from build123d import *

# Parameters (mm, degrees)
F1_DEPTH = 5


with BuildPart() as f1:
    # F0 (on Top) → F1 (new body)
    with BuildSketch(Plane.XY):
        with BuildLine():
            Line((23.528581, 23.329832), (-26.471419, 23.329832))
            Line((-26.471419, 23.329832), (-26.471419, 1.829832))
            ThreePointArc((-26.471419, 1.829832), (-26.032079, 0.769172), (-24.971419, 0.329832))
            Line((-24.971419, 0.329832), (-24.25406, 0.329832))
            ThreePointArc((-24.25406, 0.329832), (-23.614457, 0.473031), (-23.096976, 0.875286))
            ThreePointArc((-23.096976, 0.875286), (-16.011419, -1.670168), (-23.096976, -4.215623))
            ThreePointArc((-23.096976, -4.215623), (-23.614457, -3.813367), (-24.25406, -3.670168))
            Line((-24.25406, -3.670168), (-24.971419, -3.670168))
            ThreePointArc((-24.971419, -3.670168), (-26.032079, -4.109508), (-26.471419, -5.170168))
            Line((-26.471419, -5.170168), (-26.471419, -26.670168))
            Line((-26.471419, -26.670168), (23.528581, -26.670168))
            Line((23.528581, -26.670168), (23.528581, -5.170168))
            ThreePointArc((23.528581, -5.170168), (23.967921, -4.109508), (25.028581, -3.670168))
            Line((25.028581, -3.670168), (25.76043, -3.670168))
            ThreePointArc((25.76043, -3.670168), (26.39723, -3.812049), (26.913562, -4.210853))
            ThreePointArc((26.913562, -4.210853), (30.318704, -5.639032), (33.442526, -3.670168))
            ThreePointArc((33.442526, -3.670168), (33.98853, -1.672874), (33.462722, 0.329832))
            ThreePointArc((33.462722, 0.329832), (30.322397, 2.333369), (26.892574, 0.880056))
            ThreePointArc((26.892574, 0.880056), (26.373965, 0.47435), (25.731572, 0.329832))
            Line((25.731572, 0.329832), (25.028581, 0.329832))
            ThreePointArc((25.028581, 0.329832), (23.967921, 0.769172), (23.528581, 1.829832))
            Line((23.528581, 1.829832), (23.528581, 23.329832))
        make_face()
    extrude(amount=F1_DEPTH)


solid = f1.part
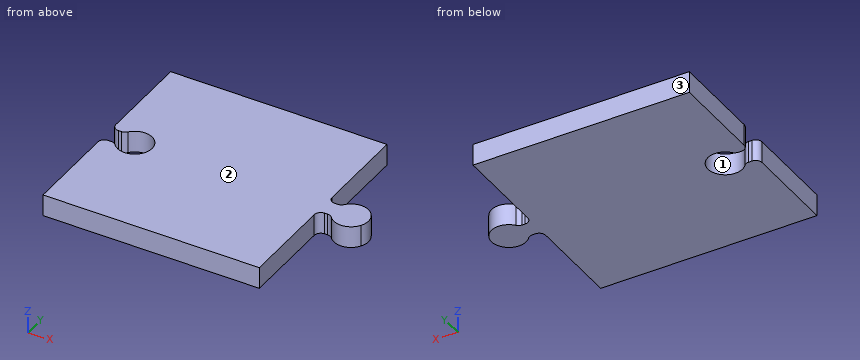
Could you check a few things on this model? Use its own coordinates, in mm. Face numbers are marked on the shaded views. Round coordinates to 2 decimals unless told otherwise and drop trailing zeros. Write each loop counter-clockwise with the first axis right and the second up, starting at its lowest first coordinate (ties: lowest second). Pieces come first, ordered by that corner, then holes. Notation, with made-up numbers: (62.5, -8) - (110.5, -8) arc R26 cw to (110.5, 22) - close; hole circle Ø1 at (2, 23). An arc over 180 degrees is marked (long way). Put each result on its own line as item: value. Start each with the question number.
(1) I want a section at B-B, the plane y = -15.5. Please give me the cut outline in (x, z), plus the area to 3 significant figures.
(2) I want a section at C-C, the plane y = -1. Please give me the cut outline in (x, z), plus the area to 3 significant figures.
(3) I want a section at A-A, the plane z = 2.65. Please give me the cut outline in (x, y), plus the area to 3 significant figures.
(4) I need wall thicknesses on probe 1 along X at (y, z) = (-5, 1.75); probe 2 along X at (y, z) = (-14, 3.3); probe 3 along X at (y, z) = (0.5, 1.9). Which ranges of each line are inside material? Lowest first, please.
(5) Thinking about a two-plate mould opening in Y: for the marked faces 1, 2 and 3, which applies, released by +Y, released by -Y, zero draft, split by the parting line, or undercut?
(6) Will these pins go through, and if not, where does the flat tip stop? pin 1 (0.8 mm diameter, centred on x = 25.5, z = 2, fed in from +Y); pin 2 (10 mm diameter, centred on x = -5.5, y = 12, fed in from -Z); pin 3 (7 mm diameter, centred on x = -20.01, y = -1.67, fed in from -Z); pin 4 (3 mm diameter, centred on y = -11, z = 4, fed in from +X).
Here are the results:
1. outline: (-26.47, 0) - (23.53, 0) - (23.53, 5) - (-26.47, 5) - close
1. area: 250 mm^2
2. outline: (-16.07, 0) - (33.93, 0) - (33.93, 5) - (-16.07, 5) - close
2. area: 250 mm^2
3. outline: (-26.47, -26.67) - (23.53, -26.67) - (23.53, -5.17) arc R1.5 cw to (25.03, -3.67) - (25.76, -3.67) arc R1.5 cw to (26.91, -4.21) arc R4 ccw to (33.44, -3.67) arc R4 ccw to (33.46, 0.33) arc R4 ccw to (26.89, 0.88) arc R1.5 cw to (25.73, 0.33) - (25.03, 0.33) arc R1.5 cw to (23.53, 1.83) - (23.53, 23.33) - (-26.47, 23.33) - (-26.47, 1.83) arc R1.5 ccw to (-24.97, 0.33) - (-24.25, 0.33) arc R1.5 ccw to (-23.1, 0.88) arc R4 cw (long way) to (-23.1, -4.22) arc R1.5 ccw to (-24.25, -3.67) - (-24.97, -3.67) arc R1.5 ccw to (-26.47, -5.17) - close
3. area: 2,500 mm^2
4. probe 1: x = -26.46 to -22.23, -17.8 to 23.54, 27.8 to 32.18
4. probe 2: x = -26.47 to 23.53
4. probe 3: x = -25.67 to -23.56, -16.65 to 24.33, 26.43 to 33.36
5. face 1: undercut
5. face 2: zero draft
5. face 3: released by +Y
6. pin 1: stops at y = 0.34
6. pin 2: stops at z = 0
6. pin 3: passes through
6. pin 4: stops at x = 23.53
